Job drawing, mm, ordinate dimensions from the low corner. One solid piece. A direction names the side the tool comes from. Coordinates: 2 decimals unless noted, no trailing zeros. Order: outer loops, then holes, each group sorted by start corner. A loop starts at its lowest first (then second) coordinate and runs counter-clockwise, first axis right, second up. Notation, with made-up numbers: (-19, -28.75) -> (14, -28.75) arc R13 ccw to (14, -7.75) -> close; hole circle Ø2 at (6, 68.25). An arc over 180 degrees is marked (long way). Use CSV: the item, a comma, the result in double quotes. Start each with the question number.
(1) Pin check, flat tips, straight feed: pin 1 Ø1 at (x, y) = (655, 180.5) entering from -Z; pin 2 Ø3 at (x, y) = (257.5, 415) entering from -Z; pin 3 Ø6 at (y, z) = (117, 1151.5) entering from -X. Stop position of each tip, or through.
(2) Probe L1, parallel to Z at x = 432.5, y = 200; L2, parallel to X at y = 454, z = 1006.5; L3, parallel to X at y = 514, z = 1067. List the from-to ranges inside material, lowest first.
(3) Cut at C-C on x = 111. Write the cut outline in (y, z), plus the area to 3 significant figures.
(4) Pull direction X, two halves, no side cores. Call the marked faces 4, 5 and 6: pulls with the +X half, pulls with the -X half, needs draft (parallel to the pull), parting line crosses it, or undercut.
(5) Tool access for the marked faces 1, 2 and 3: list every direction of +Z, -Z, +X, -X, +Y, -Y with a clear straight run to the whole face (end or side of a thin tool).
(6) Cut at D-D on x = 1205.5. Write the cut outline in (y, z).
(7) Cut at A-A on y = 256. Write the cut outline in (x, z), plus the area to 4 significant figures.
(8) Cut at B-B on z = 347. Write the cut outline in (x, y).
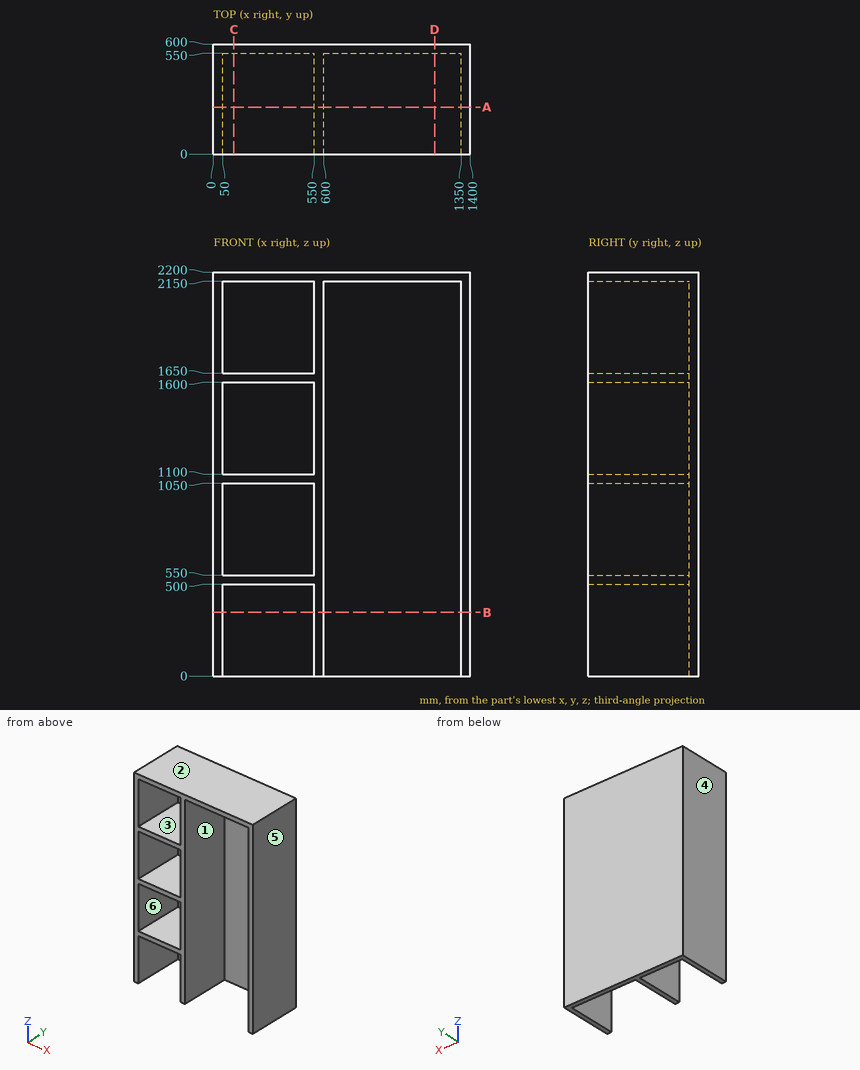
Outcome:
1,pin 1,"z = 2150"
1,pin 2,"z = 500"
1,pin 3,"x = 0"
2,L1,"500 to 550, 1050 to 1100, 1600 to 1650, 2150 to 2200"
2,L2,"0 to 50, 550 to 600, 1350 to 1400"
2,L3,"0 to 600, 1350 to 1400"
3,outline,"(0, 500) -> (550, 500) -> (550, 0) -> (600, 0) -> (600, 2200) -> (0, 2200) -> (0, 2150) -> (550, 2150) -> (550, 1650) -> (0, 1650) -> (0, 1600) -> (550, 1600) -> (550, 1100) -> (0, 1100) -> (0, 1050) -> (550, 1050) -> (550, 550) -> (0, 550) -> close"
3,area,"220,000 mm2"
4,face 4,"pulls with the -X half"
4,face 5,"pulls with the +X half"
4,face 6,"undercut"
5,face 1,"-Z, -Y"
5,face 2,"+Z, +X, -X, +Y, -Y"
5,face 3,"-Y"
6,outline,"(0, 2150) -> (550, 2150) -> (550, 0) -> (600, 0) -> (600, 2200) -> (0, 2200) -> close"
7,outline,"(0, 0) -> (50, 0) -> (50, 500) -> (550, 500) -> (550, 0) -> (600, 0) -> (600, 2150) -> (1350, 2150) -> (1350, 0) -> (1400, 0) -> (1400, 2200) -> (0, 2200) -> close; hole (50, 550) -> (550, 550) -> (550, 1050) -> (50, 1050) -> close; hole (50, 1100) -> (550, 1100) -> (550, 1600) -> (50, 1600) -> close; hole (50, 1650) -> (550, 1650) -> (550, 2150) -> (50, 2150) -> close"
7,area,"467,500 mm2"
8,outline,"(0, 0) -> (50, 0) -> (50, 550) -> (550, 550) -> (550, 0) -> (600, 0) -> (600, 550) -> (1350, 550) -> (1350, 0) -> (1400, 0) -> (1400, 600) -> (0, 600) -> close"
